```python
from build123d import *

# Parameters (mm, degrees)
BOSS_EXTRUDE1_DEPTH = 3.75


with BuildPart() as part:
    # Sketch1 → Revolve1 (revolve)
    with BuildSketch(Plane.XY, mode=Mode.PRIVATE) as revolve1_sk:
        Polygon((0, 0), (0, 1.5), (-29.75, 1.5), (-30, 1.25), (-30, 0), align=None)
    revolve(revolve1_sk.sketch.rotate(Axis((-30, 0, 0), (1, 0, 0)), 90), axis=Axis((-30, 0, 0), (1, 0, 0)))

    # Sketch2 → Boss-Extrude1 (add)
    with BuildSketch(Plane(origin=(0, 0, 0), x_dir=(0, 0, -1), z_dir=(1, 0, 0))):
        Polygon((-1.58771324, 2.75), (0, 2.75), (1.58771324, 2.75), (2.38156986, 1.375), (3.175426481, 0), (2.38156986, -1.375), (1.58771324, -2.75), (0, -2.75), (-1.58771324, -2.75), (-2.38156986, -1.375), (-3.175426481, 0), (-2.38156986, 1.375), align=None)
    extrude(amount=BOSS_EXTRUDE1_DEPTH)

    # Sketch3 → Cut-Revolve3 (revolve, cut)
    with BuildSketch(Plane.XY, mode=Mode.PRIVATE) as cut_revolve3_sk:
        Polygon((4, -2.25), (3.5, -2.75), (2.25, -4), (5.25, -4), (5.25, -1), align=None)
    revolve(cut_revolve3_sk.sketch.rotate(Axis((0, 0, 0), (1, 0, 0)), 270), axis=Axis((0, 0, 0), (1, 0, 0)), mode=Mode.SUBTRACT)


solid = part.part
```
Geometry check sheet. Reference: the model listing, model coordinates, mm. A direction names the side the tool comes from. Round coordinates to 2 decimals unless told otherwise and drop trailing zeros. Order: outer loops, then holes, each group sorted by start corner. A loop starts at its lowest first (then second) coordinate and runs counter-clockwise, first axis right, second up. Notation, with made-up numbers: (23.5, 28.5) -> (65.5, 28.5) arc R25 cw to (65.5, 49.5) -> close; hole circle Ø4 at (-21, 66.25). An arc over 180 degrees is marked (long way). Return JSON: item names as keys, results as strings. Group by question number.
Q1. Section check A-A, the plane z = 0. Record the boundary of the cut face in (x, y), plus the area to 4 significant figures.
Q2. Tool access check on faces 1 (the flat face through (-30, 0, 0)), 2 (the cylindrical face through (-15.08, -0.45, 1.43)). Record the directions out of +Z, -Z, +X, -X, +Y, -Y that give a thin tool (end or side, any length) a straight path to the whole face; none if there is none.
Q3. Gauge pin test, flat ends, axial feed: pin 1 (1.5 mm diameter, centred on x = -22.5, y = 1, fed in from +Z); pin 2 (1 mm diameter, centred on x = -3, y = -1, fed in from -Z). Record the tip position at first contact, or that the pin passes through.
Q4. Material ranges on probe 1 along X at (y, z) = (-0.05, 1.25); probe 2 along X at (y, z) = (0.6, -2.25); probe 3 along Z at (x, y) = (-19, 0.45), recorded low to high. Write a range as from..to.
Q5. Section check B-B, the plane x = -25. Record the boundary of the cut face in (y, z), plus the area to 3 significant figures.
Numbers:
{
 "1": {"outline": "(-30, -1.25) -> (-29.75, -1.5) -> (0, -1.5) -> (0, -2.75) -> (3.5, -2.75) -> (3.75, -2.5) -> (3.75, 2.5) -> (3.5, 2.75) -> (0, 2.75) -> (0, 1.5) -> (-29.75, 1.5) -> (-30, 1.25) -> close", "area": "110.5 mm^2"},
 "2": {"face 1": "+Z, -Z, -X, +Y, -Y", "face 2": "-X"},
 "3": {"pin 1": "z = 1.48", "pin 2": "z = -1.41"},
 "4": {"probe 1": "-30..3.75", "probe 2": "0..3.75", "probe 3": "-1.43..1.43"},
 "5": {"outline": "circle Ø3 at (0, 0)", "area": "7.07 mm^2"}
}
